from build123d import *

# Parameters (mm, degrees)
F0_W     = 76.2
F0_H     = 25.4
F1_DEPTH = 5.08
F3_DEPTH = 12.7


with BuildPart() as f1:
    # F0 (on Front) → F1 (new body)
    with BuildSketch(Plane.XZ):
        Rectangle(F0_W, F0_H)
    extrude(amount=F1_DEPTH)

    # F2 (on face) → F3 (join)
    with BuildSketch(Plane.XZ.offset(5.08)):
        with BuildLine():
            ThreePointArc((-18.079832, -12.7), (-9.099576, -8.980256), (-5.379832, 0))
            ThreePointArc((-5.379832, 0), (-5.435483, 1.187617), (-5.601948, 2.364825))
            ThreePointArc((-5.601948, 2.364825), (-5.784143, 3.178999), (-6.019403, 3.979452))
            ThreePointArc((-6.019403, 3.979452), (-10.638362, 10.291478), (-18.079832, 12.7))
            ThreePointArc((-18.079832, 12.7), (-30.779832, 0), (-18.079832, -12.7))
        make_face()
        with BuildLine():
            ThreePointArc((-6.019403, 3.979452), (-5.784143, 3.178999), (-5.601948, 2.364825))
            ThreePointArc((-5.601948, 2.364825), (-0.027745, 4.54921), (5.678145, 2.736451))
            ThreePointArc((5.678145, 2.736451), (5.873958, 3.508082), (6.117731, 4.265928))
            ThreePointArc((6.117731, 4.265928), (-0.004095, 6.379128), (-6.019403, 3.979452))
        make_face()
        with BuildLine():
            ThreePointArc((6.117731, 4.265928), (5.873958, 3.508082), (5.678145, 2.736451))
            ThreePointArc((5.678145, 2.736451), (8.179253, -7.954152), (18.079832, -12.7))
            ThreePointArc((18.079832, -12.7), (27.060088, -8.980256), (30.779832, 0))
            ThreePointArc((30.779832, 0), (27.060088, 8.980256), (18.079832, 12.7))
            ThreePointArc((18.079832, 12.7), (10.761611, 10.379482), (6.117731, 4.265928))
        make_face()
    extrude(amount=F3_DEPTH)


solid = f1.part
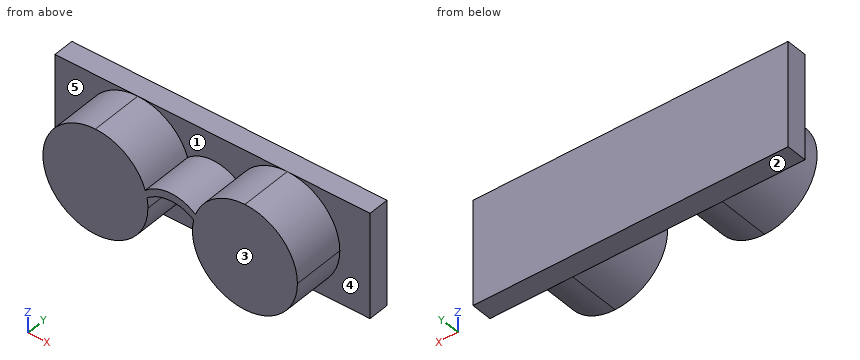
Geometry check sheet. Reference: the model listing, model coordinates, mm. Face numbers are marked on the shaded views. A direction names the side the tool comes from. Give positions to 0.01 mm unless a question says otherwise; leave off trailing zeros. Order: outer loops, then holes, each group sorted by start corner. A loop starts at its lowest first (then second) coordinate and runs counter-clockwise, first axis right, second up. Notation, with made-up numbers: (-34.75, 32.25) - (23.25, 32.25) arc R26 ccw to (23.25, 69.25) - close; hole circle Ø9 at (54, -23.5). An arc over 180 degrees is marked (long way). Answer as a JSON object with one key per item and string values.
(1) Cross-section at C-C (z = -2.75). Record the cut outline in (x, y), then the cut area to 3 significant figures.
Report:
{"outline": "(-38.1, -5.08) - (-30.48, -5.08) - (-30.48, -17.78) - (-5.68, -17.78) - (-5.68, -5.08) - (5.68, -5.08) - (5.68, -17.78) - (30.48, -17.78) - (30.48, -5.08) - (38.1, -5.08) - (38.1, 0) - (-38.1, 0) - close", "area": "1,020 mm^2"}
(2) Depth check by flat-ended pin: pin 1 Ø8 at (x, z) = (28, 1.5) entering from +Y; pin 2 Ø1.5 at (y, z) = (-11, -1) entering from +X; pin 3 Ø6 at (x, z) = (2.5, -7.5) entering from -Y; pin 4 Ø1 at (y, z) = (-14, -3) entering from +X. Enter the tip coordinate at first touch or a pass-through.
Report:
{"pin 1": "y = 0", "pin 2": "x = 30.78", "pin 3": "y = -5.08", "pin 4": "x = 30.53"}
(3) Cross-section at B-B (x = 24.5). Record the cut outline in (y, z).
Report:
{"outline": "(-17.78, -10.96) - (-5.08, -10.96) - (-5.08, -12.7) - (0, -12.7) - (0, 12.7) - (-5.08, 12.7) - (-5.08, 10.96) - (-17.78, 10.96) - close"}
(4) Material ranges on line 1 (Y direction, x = 33, z = 3.5); line 2 (X direction, y = -14.25, z = -11.25); line 3 (X direction, y = -7.25, z = -1.25), recorded low to high.
Report:
{"line 1": "-5.08 to 0", "line 2": "-23.97 to -12.19, 12.19 to 23.97", "line 3": "-30.72 to -5.44, 5.44 to 30.72"}
(5) Tool access check on the marked faces 1, 2, 3, 4 and 5. Record the directions out of +Z, -Z, +X, -X, +Y, -Y that give a thin tool (end or side, any length) a straight path to the whole face; none if there is none.
Report:
{"face 1": "+Z, -Y", "face 2": "-Z, +X, -X, +Y, -Y", "face 3": "+Z, -Z, +X, -X, -Y", "face 4": "+X, -Y", "face 5": "-X, -Y"}
(6) Cross-section at D-D (z = 10.25). Record the cut outline in (x, y).
Report:
{"outline": "(-38.1, -5.08) - (-25.58, -5.08) - (-25.58, -17.78) - (-10.58, -17.78) - (-10.58, -5.08) - (10.58, -5.08) - (10.58, -17.78) - (25.58, -17.78) - (25.58, -5.08) - (38.1, -5.08) - (38.1, 0) - (-38.1, 0) - close"}
(7) Cross-section at A-A (y = -7.25). Record the cut outline in (x, z).
Report:
{"outline": "(-18.08, 12.7) arc R12.7 ccw (long way) to (-5.38, 0) arc R12.7 ccw to (-5.6, 2.36) arc R8.96 cw to (5.68, 2.74) arc R12.7 ccw (long way) to (18.08, 12.7) arc R12.7 ccw to (6.12, 4.27) arc R9.29 ccw to (-6.02, 3.98) arc R12.7 ccw to start"}
